```python
from build123d import *

# Parameters (mm, degrees)
SKETCH145_R     = 1.6
PAD079_DEPTH    = 3
CHAMFER051_SIZE = 2
FILLET047_R     = 2
SKETCH_W        = 38
SKETCH_H        = 10
POCKET_DEPTH    = 3.001
CHAMFER_SIZE    = 2


with BuildPart() as part:
    # Sketch145 → Pad079 (new body)
    with BuildSketch(Plane.XY):
        with BuildLine():
            Line((-18, 55), (20, 55))
            Line((20, 55), (20, -10))
            Line((20, -10), (10, -10))
            ThreePointArc((10, -10), (9.707107, -9.292893), (9, -9))
            Line((5, -9), (9, -9))
            ThreePointArc((5, -9), (4.292893, -9.292893), (4, -10))
            Line((4, -10), (-8, -10))
            ThreePointArc((-8, -10), (-8.292893, -9.292893), (-9, -9))
            Line((-13, -9), (-9, -9))
            ThreePointArc((-13, -9), (-13.707107, -9.292893), (-14, -10))
            Line((-14, -10), (-18, -10))
            Line((-18, -10), (-18, 55))
        make_face()
        with Locations((15.5, 25)):
            Circle(SKETCH145_R, mode=Mode.SUBTRACT)
        with Locations((15.5, 33)):
            Circle(SKETCH145_R, mode=Mode.SUBTRACT)
        with Locations((5.999998, 51.999985)):
            Circle(SKETCH145_R, mode=Mode.SUBTRACT)
        with Locations((-7.000002, 51.999985)):
            Circle(SKETCH145_R, mode=Mode.SUBTRACT)
        with Locations((-7.000002, 2.999985)):
            Circle(SKETCH145_R, mode=Mode.SUBTRACT)
        with Locations((5.999998, 2.999985)):
            Circle(SKETCH145_R, mode=Mode.SUBTRACT)
        with BuildLine():
            ThreePointArc((-13, -2), (-14, -3), (-13, -4))
            Line((-13, -4), (-9, -4))
            ThreePointArc((-9, -4), (-8, -3), (-9, -2))
            Line((-13, -2), (-9, -2))
        make_face(mode=Mode.SUBTRACT)
        with BuildLine():
            ThreePointArc((5, -2), (4, -3), (5, -4))
            Line((5, -4), (9, -4))
            ThreePointArc((9, -4), (10, -3), (9, -2))
            Line((5, -2), (9, -2))
        make_face(mode=Mode.SUBTRACT)
    extrude(amount=PAD079_DEPTH)

    # Chamfer051
    chamfer051_edges = [part.edges().sort_by_distance(p)[0] for p in [
        (-18, 55, 1.5),
        (20, 55, 1.5),
        (20, -10, 1.5),
        (-18, -10, 1.5),
    ]]
    chamfer(chamfer051_edges, length=CHAMFER051_SIZE)

    # Fillet047
    fillet047_edges = [part.edges().sort_by_distance(p)[0] for p in [
        (-14, -10, 1.5),
        (-8, -10, 1.5),
        (4, -10, 1.5),
        (10, -10, 1.5),
    ]]
    fillet(fillet047_edges, radius=FILLET047_R)

    # Sketch → Pocket (cut, through all)
    with BuildSketch(Plane.XY):
        with Locations((1, -5)):
            Rectangle(SKETCH_W, SKETCH_H)
    extrude(amount=POCKET_DEPTH, mode=Mode.SUBTRACT)

    # Chamfer
    chamfer_edges = [part.edges().sort_by_distance(p)[0] for p in [
        (-18, 0, 1.5),
        (20, 0, 1.5),
    ]]
    chamfer(chamfer_edges, length=CHAMFER_SIZE)


with BuildPart() as part_1:
    # Body067 placement: moved
    add(part.part.moved(Location((0, -2.3e-05, 33.499985))))


solid = part_1.part
```
Verification items for the finished model (mm, model axes). Round coordinates to 2 decimals unless told otherwise and drop trailing zeros. Order: outer loops, then holes, each group sorted by start corner. A loop starts at its lowest first (then second) coordinate and runs counter-clockwise, first axis right, second up. Notation, with made-up numbers: (30.25, 32) - (48.25, 32) arc R13 cw to (48.25, 45) - close; hole circle Ø5 at (68, -11.5). An arc over 180 degrees is marked (long way). Use CSV: the item, a comma, the result in double quotes. Start each with the question number.
1) Mould release check, pull along X, two halves, no side actions. Record for faces 1 (the cylindrical face through (-6.26, 50.58, 34.98)), 2 (the flat face through (19, 54, 35)), 3 (the flat face through (-17, 1, 35)): +X half, -X half, draft (parallel to the pull), parting line (faces both ways), or undercut.
2) Section check C-C, the plane x = -8. Record the cut outline in (y, z).
3) Section check B-B, the plane z = 35.2. Record the cut outline in (x, y), plus the area to 3 significant figures.
4) Section check A-A, the plane x = 15.5. Record the cut outline in (y, z).
5) Thickness scan on L1, parallel to Y at x = 15.5, z = 35.8; L2, parallel to Y at x = 6, z = 35.45; L3, parallel to X at y = 32, z = 35.6. Record the ranges inside material, lowest first.
Answers:
1,face 1,"undercut"
1,face 2,"+X half"
1,face 3,"-X half"
2,outline,"(0, 33.5) - (1.75, 33.5) - (1.75, 36.5) - (0, 36.5) - close; (4.25, 33.5) - (50.75, 33.5) - (50.75, 36.5) - (4.25, 36.5) - close; (53.25, 33.5) - (55, 33.5) - (55, 36.5) - (53.25, 36.5) - close"
3,outline,"(-18, 2) - (-16, 0) - (18, 0) - (20, 2) - (20, 53) - (18, 55) - (-16, 55) - (-18, 53) - close; hole circle Ø3.2 at (-7, 3); hole circle Ø3.2 at (-7, 52); hole circle Ø3.2 at (6, 3); hole circle Ø3.2 at (6, 52); hole circle Ø3.2 at (15.5, 25); hole circle Ø3.2 at (15.5, 33)"
3,area,"2,030 mm²"
4,outline,"(0, 33.5) - (23.4, 33.5) - (23.4, 36.5) - (0, 36.5) - close; (26.6, 33.5) - (31.4, 33.5) - (31.4, 36.5) - (26.6, 36.5) - close; (34.6, 33.5) - (55, 33.5) - (55, 36.5) - (34.6, 36.5) - close"
5,L1,"y = 0 to 23.4, 26.6 to 31.4, 34.6 to 55"
5,L2,"y = 0 to 1.4, 4.6 to 50.4, 53.6 to 55"
5,L3,"x = -18 to 14.25, 16.75 to 20"
